```python
from build123d import *

# Parameters (mm, degrees)
SKETCH1_W                       = 40.7
SKETCH1_H                       = 39.5
BOSS_EXTRUDE1_DEPTH             = 10
SKETCH2_W                       = 2.5
SKETCH2_H                       = 20
BOSS_EXTRUDE2_DEPTH             = 7
BOSS_EXTRUDE5_DEPTH             = 0.5
CUT_EXTRUDE1_DEPTH              = 34.3
SKETCH4_R                       = 6.57
BOSS_EXTRUDE3_DEPTH             = 1.5
SKETCH5_R                       = 3
BOSS_EXTRUDE4_DEPTH             = 4.2
M3X0_5_TAPPED_HOLE1_D           = 2.5
M3X0_5_TAPPED_HOLE1_DEPTH       = 5
M3X0_5_TAPPED_HOLE1_CSINK_D     = 3.05
M3X0_5_TAPPED_HOLE1_CSINK_ANGLE = 90
M3X0_5_TAPPED_HOLE1_TIP         = 0.751075774


with BuildPart() as part:
    # Sketch1 → Boss-Extrude1 (new body, symmetric)
    with BuildSketch(Plane(origin=(0, 0, 0), x_dir=(1, 0, 0), z_dir=(0, 1, 0))):
        Rectangle(SKETCH1_W, SKETCH1_H)
    extrude(amount=BOSS_EXTRUDE1_DEPTH, both=True)

    # Sketch2 → Boss-Extrude2 (add)
    with BuildSketch(Plane(origin=(20.35, 0, 0), x_dir=(0, 0, -1), z_dir=(1, 0, 0))):
        with Locations((12.3, 0)):
            Rectangle(SKETCH2_W, SKETCH2_H)
    boss_extrude2 = extrude(amount=BOSS_EXTRUDE2_DEPTH)

    # Sketch9 → Boss-Extrude5 (add, symmetric)
    with BuildSketch(Plane(origin=(0, 0, 0), x_dir=(1, 0, 0), z_dir=(0, 1, 0))):
        Polygon((20.35, 13.55), (20.35, 14.65), (27.35, 13.55), align=None)
    boss_extrude5 = extrude(amount=BOSS_EXTRUDE5_DEPTH, both=True)

    # Mirror1: Boss-Extrude2, Boss-Extrude5 across plane
    add(boss_extrude2.mirror(Plane(origin=(0, 0, 0), x_dir=(0, 0, 1), z_dir=(1, 0, 0))))
    add(boss_extrude5.mirror(Plane(origin=(0, 0, 0), x_dir=(0, 0, 1), z_dir=(1, 0, 0))))

    # Sketch3 → Cut-Extrude1 (cut, through all)
    with BuildSketch(Plane(origin=(0, 0, -13.55), x_dir=(-1, 0, 0), z_dir=(0, 0, -1))):
        with BuildLine():
            Line((-26.243988636, 6.675), (-27.35, 6.675))
            Line((-27.35, 6.675), (-27.35, 4.525))
            Line((-27.35, 4.525), (-26.243988636, 4.525))
            ThreePointArc((-26.243988636, 4.525), (-22.34, 5.6), (-26.243988636, 6.675))
        make_face()
        with BuildLine():
            Line((26.243988636, 6.675), (27.35, 6.675))
            Line((27.35, 6.675), (27.35, 4.525))
            Line((27.35, 4.525), (26.243988636, 4.525))
            ThreePointArc((26.243988636, 4.525), (22.34, 5.6), (26.243988636, 6.675))
        make_face()
    cut_extrude1 = extrude(amount=-CUT_EXTRUDE1_DEPTH, mode=Mode.SUBTRACT)

    # Mirror2: Cut-Extrude1 across plane
    add(cut_extrude1.mirror(Plane.ZX), mode=Mode.SUBTRACT)

    # Sketch4 → Boss-Extrude3 (add)
    with BuildSketch(Plane(origin=(0, 0, -19.75), x_dir=(-1, 0, 0), z_dir=(0, 0, -1))):
        with Locations((-10.62, 0)):
            Circle(SKETCH4_R)
    extrude(amount=BOSS_EXTRUDE3_DEPTH)

    # Sketch5 → Boss-Extrude4 (add)
    with BuildSketch(Plane(origin=(0, 0, -21.25), x_dir=(-1, 0, 0), z_dir=(0, 0, -1))):
        with Locations((-10.62, 0)):
            Circle(SKETCH5_R)
    extrude(amount=BOSS_EXTRUDE4_DEPTH)

    # M3x0.5 Tapped Hole1
    with Locations(Plane(origin=(0, 0, -25.45), x_dir=(-1, 0, 0), z_dir=(0, 0, -1))):
        with Locations((-10.62, 0)):
            CounterSinkHole(M3X0_5_TAPPED_HOLE1_D / 2, M3X0_5_TAPPED_HOLE1_CSINK_D / 2, depth=M3X0_5_TAPPED_HOLE1_DEPTH, counter_sink_angle=M3X0_5_TAPPED_HOLE1_CSINK_ANGLE)
            with Locations((0, 0, -(M3X0_5_TAPPED_HOLE1_DEPTH + M3X0_5_TAPPED_HOLE1_TIP / 2))):  # 118° drill point
                Cone(0, M3X0_5_TAPPED_HOLE1_D / 2, M3X0_5_TAPPED_HOLE1_TIP, mode=Mode.SUBTRACT)


solid = part.part
```
Read the model definition and answer for the solid it produces. Units are mm, in the model's axes. A direction names the side the tool comes from. Coordinates: 2 decimals unless noted, no trailing zeros. Loops run counter-clockwise (first coordinate to the right, second up) from the corner with the lowest first, then second, coordinate; pieces in that order, holes last. Notation, with made-up numbers: (-35.75, 19) - (11.25, 19) arc R8 cw to (11.25, 31) - close; hole circle Ø5 at (70, 39.5). An arc over 180 degrees is marked (long way). Answer in a Markdown table with one row per item.
1. Given pin 1 (3 mm diameter, centred on y = 4.5, z = 10, fed in from +X); pin 2 (1.5 mm diameter, centred on x = -3.5, y = 3, fed in from -Z); pin 3 (5 mm diameter, centred on y = -5, z = -11, fed in from -X); pin 4 (5.5 mm diameter, centred on x = -25, y = 3.5, fed in from -Z), each flat-ended and moving along its own axis, determine where each tip first touches the part or whether it passes through.
Conclusion:
| item | result |
|---|---|
| pin 1 | stops at x = 20.35 |
| pin 2 | stops at z = -19.75 |
| pin 3 | stops at x = -27.35 |
| pin 4 | stops at z = -13.55 |
2. Find section C-C, the plane y = 5.6. Write down the section's boundary in (x, z).
Conclusion:
| item | result |
|---|---|
| outline | (-22.34, -13.55) - (-20.35, -13.55) - (-20.35, -19.75) - (7.18, -19.75) - (7.18, -21.25) - (14.06, -21.25) - (14.06, -19.75) - (20.35, -19.75) - (20.35, -13.55) - (22.34, -13.55) - (22.34, -11.05) - (20.35, -11.05) - (20.35, 19.75) - (-20.35, 19.75) - (-20.35, -11.05) - (-22.34, -11.05) - close |
3. Find section D-D, the plane x = 3. Write down the section's boundary in (y, z).
Conclusion:
| item | result |
|---|---|
| outline | (-10, -19.75) - (10, -19.75) - (10, 19.75) - (-10, 19.75) - close |
4. Find section B-B, the plane z = -5.5. Write down the section's boundary in (x, y), then the cut area to 3 significant figures.
Conclusion:
| item | result |
|---|---|
| outline | (-20.35, -10) - (20.35, -10) - (20.35, 10) - (-20.35, 10) - close |
| area | 814 mm² |
5. Find section A-A, the plane x = -24. Write down the section's boundary in (y, z).
Conclusion:
| item | result |
|---|---|
| outline | (-10, -13.55) - (-7.65, -13.55) - (-7.65, -11.05) - (-10, -11.05) - close; (-3.55, -13.55) - (-0.5, -13.55) - (-0.5, -14.08) - (0.5, -14.08) - (0.5, -13.55) - (3.55, -13.55) - (3.55, -11.05) - (-3.55, -11.05) - close; (7.65, -13.55) - (10, -13.55) - (10, -11.05) - (7.65, -11.05) - close |
6. Determine the mould class of faces 1 (the face through (-22, 5, -13.55)), 2 (the face through (27.35, 0, -12)), 3 (the face through (-22.34, -5.52, -12.32)), 4 (the face through (-27.35, 8, -12)) for opening direction X: +X half, -X half, draft (parallel to the pull), parting line (faces both ways), or undercut.
Conclusion:
| item | result |
|---|---|
| face 1 | draft |
| face 2 | +X half |
| face 3 | undercut |
| face 4 | -X half |
7. Which of the six approach directions +Z, -Z, +X, -X, +Y, -Y give full straight-line access (tool end or side, diameter ignored) to faces 5 (the face through (17.184, 0.289, -20.49)), 6 (the face through (27, 6.675, -12)), 7 (the face through (-22, -5, -13.55)), 8 (the face through (24, 0, -11.05)), 9 (the face through (22, 5, -13.55))?
Conclusion:
| item | result |
|---|---|
| face 5 | -Z |
| face 6 | +Z, -Z, +X |
| face 7 | -Z, -X, -Y |
| face 8 | +Z, +X, +Y, -Y |
| face 9 | -Z, +X, +Y |
8. Straight lines are drawn through the part: line 1 (Y direction, x = 24.44, z = -12.05); line 2 (X direction, y = 3, z = -2.5); line 3 (X direction, y = 5.6, z = -11.65). For each, find the intervals that lie inside material, in ascending order.
Conclusion:
| item | result |
|---|---|
| line 1 | y = -10 to -7.7, -3.5 to 3.5, 7.7 to 10 |
| line 2 | x = -20.35 to 20.35 |
| line 3 | x = -22.34 to 22.34 |
